Part model, mm, in its own coordinate system. Face numbers are marked on the shaded views. A direction names the side the tool comes from. Round coordinates to 2 decimals unless told otherwise and drop trailing zeros. Loops run counter-clockwise (first coordinate to the right, second up) from the corner with the lowest first, then second, coordinate; pieces in that order, holes last. Notation, with made-up numbers: (87, 34.25) - (124, 34.25) arc R29 cw to (124, 60.25) - close; hole circle Ø2 at (78.25, 28.5). An arc over 180 degrees is marked (long way). Write each question's results on one line, items separated by ' | '. Start each with the question number.
(1) Cut at D-D, the plane x = -40.5. List the corners of the cut face in (y, z) (3 decimals), then the cut area to 3 significant figures.
(2) Drill centre lines: L1, parallel to X at y = 23.5, z = 11; L2, parallel to Y at x = -29, z = 13.25; L3, parallel to X at y = -0.5, z = 14.25. Where is each one in solid material? Low to high.
(3) Mould opens along Y. For the marked faces 6, 7, 8 and 9 say: released by +Y, released by -Y, zero draft, split by the parting line, or undercut.
(4) Cut at B-B, the plane x = -24.5. List the corners of the cut face in (y, z).
(5) Cut at A-A, the plane y = 8. List the corners of the cut face in (x, z).
(6) Cut at C-C, the plane z = 16.5. List the corners of the cut face in (x, y), then the cut area to 3 significant figures.
(7) Tool access for the marked faces 1, 2, 3, 4 and 5: list every direction of +Z, -Z, +X, -X, +Y, -Y with a clear straight run to the whole face (end or side of a thin tool).
(8) Flat gauge pins, fed straight in: P1, Ø4, axis at x = -40.5, z = 17.5, coming from the +Y side; P2, Ø3, axis at x = -43.5, z = 11.5, coming from the -Y side; P3, Ø1.1, axis at x = 1.5, z = 13.5, coming from the -Y side; P4, Ø3, axis at y = 44, z = 11.5, coming from the +X side. Where does each tip first touch, or does it go through?
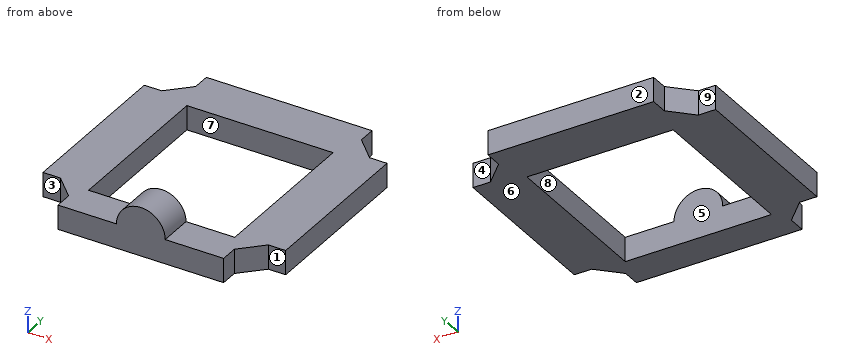
Autodesk Inventor part; units mm, degrees
ref_plane "Work Plane1" through (0, 0, 10) normal (0, 0, 1) x (1, 0, 0)
ref_plane "YZ Plane" through (0, 0, 0) normal (1, 0, 0) x (0, 1, 0)
ref_plane "XZ Plane" through (0, 0, 0) normal (0, 1, 0) x (-1, 0, 0)
ref_plane "Work Plane1" through (0, 0, 10) normal (0, 0, 1) x (1, 0, 0)
sketch "Sketch1" plane through (0, 0, 10) normal (0, 0, 1) x (1, 0, 0)
  line L0 (-4.0299, -0.3538) -> (-2.2322, 1.4439) construction
  arc A0 (-1.4439, 2.2322) -> (-2.2322, 1.4439) centre (-0.9299, 0.9299) ccw construction
  line L1 (-1.4439, 2.2322) -> (0.3538, 4.0299) construction
  line L2 (-37.8299, 42.2137) -> (-37.8299, 45.8299) construction
  line L3 (-37.8299, 45.8299) -> (-4.0299, 45.8299) construction
  line L4 (-4.0299, 45.8299) -> (-4.0299, 42.2137) construction
  line L5 (-4.0299, 4.0299) -> (0.3538, 4.0299)
  circle A1 centre (-20.9299, 20.9299) radius 17.5
  line L6 (-20.9299, 58.9723) -> (17.1124, 20.9299) construction
  line L7 (17.1124, 20.9299) -> (-20.9299, -17.1124) construction
  line L8 (-20.9299, -17.1124) -> (-58.9723, 20.9299) construction
  line L9 (-58.9723, 20.9299) -> (-20.9299, 58.9723) construction
  line L10 (-20.9299, 58.9723) -> (-20.9299, -17.1124) construction
  line L11 (17.1124, 20.9299) -> (-58.9723, 20.9299) construction
  line L12 (-20.9299, 58.9723) -> (32.8701, 58.9723) construction
  line L13 (-43.4299, 43.4299) -> (1.5701, 43.4299) construction
  line L14 (1.5701, 43.4299) -> (1.5701, -1.5701) construction
  line L15 (1.5701, -1.5701) -> (-43.4299, -1.5701) construction
  line L16 (-43.4299, -1.5701) -> (-43.4299, 43.4299) construction
  line L17 (-43.4299, 43.4299) -> (1.5701, -1.5701) construction
  line L18 (1.5701, 43.4299) -> (-43.4299, -1.5701) construction
  line L19 (-43.4299, 5.3876) -> (-43.4299, 36.4723)
  line L20 (-43.4299, 36.4723) -> (-36.4723, 43.4299)
  line L21 (-36.4723, 43.4299) -> (-5.3876, 43.4299)
  line L22 (-5.3876, 43.4299) -> (1.5701, 36.4723)
  line L23 (1.5701, 36.4723) -> (1.5701, 5.3876)
  line L24 (1.5701, 5.3876) -> (-5.3876, -1.5701)
  line L25 (-5.3876, -1.5701) -> (-36.4723, -1.5701)
  line L26 (-36.4723, -1.5701) -> (-43.4299, 5.3876)
  line L27 (-4.0299, 42.2137) -> (-37.8299, 42.2137)
  line L28 (-4.0299, -0.3538) -> (-4.0299, 4.0299)
  circle A2 centre (-20.9299, 20.9299) radius 0.4266
  point P0 (-37.8299, 4.0299)
  dimension "d18" = 53.8
  dimension "d19" = 45
  dimension "d20" = 53.8
  dimension "d21" = 45
  dimension "d22" = 45
extrude "Extrusion1" add sketch "Sketch1" along normal blind 5 contours L28 L24 L25 L26 L19 L20 L27 L22 L23 L5 | L5 L24 L28 | L27 L20 L21 L22 | A1
sketch "Sketch3" plane through (0, 0, 10) normal (0, 0, -1) x (-1, 0, 0)
  line L0 (37.8299, -0.4701) -> (37.8299, 4.0299) construction
  line L1 (4.0299, 4.0299) -> (4.0299, -0.4701) construction
  line L2 (37.8299, -0.4701) -> (37.8299, 1.1886) construction
  line L3 (4.0299, -3.9701) -> (4.0299, -0.3538) construction
  line L4 (45.8299, 4.0299) -> (42.2137, 4.0299) construction
  line L5 (-0.3538, 4.0299) -> (-3.9701, 4.0299) construction
  line L6 (-3.9701, 37.8299) -> (-0.3538, 37.8299) construction
  line L7 (4.0299, 42.2137) -> (4.0299, 45.8299) construction
  line L8 (37.8299, 45.8299) -> (37.8299, 42.2137) construction
  line L9 (42.2137, 37.8299) -> (45.8299, 37.8299) construction
  line L10 (37.8299, 37.7299) -> (45.8299, 37.7299)
  line L11 (45.8299, 37.7299) -> (45.8299, 4.1299)
  line L12 (45.8299, 4.1299) -> (37.8299, 4.1299)
  line L13 (37.8299, 4.1299) -> (37.8299, 37.7299)
  line L14 (37.7299, 4.0299) -> (4.1299, 4.0299)
  line L15 (4.1299, 4.0299) -> (4.1299, -3.9701)
  line L16 (4.1299, -3.9701) -> (37.7299, -3.9701)
  line L17 (37.7299, -3.9701) -> (37.7299, 4.0299)
  line L18 (4.0299, 4.1299) -> (-3.9701, 4.1299)
  line L19 (-3.9701, 4.1299) -> (-3.9701, 37.7299)
  line L20 (-3.9701, 37.7299) -> (4.0299, 37.7299)
  line L21 (4.0299, 37.7299) -> (4.0299, 4.1299)
  line L22 (4.1299, 37.8299) -> (37.7299, 37.8299)
  line L23 (37.7299, 37.8299) -> (37.7299, 45.8299)
  line L24 (37.7299, 45.8299) -> (4.1299, 45.8299)
  line L25 (4.1299, 45.8299) -> (4.1299, 37.8299)
  point P0 (0, 0)
  dimension "d23" = 0.1
  dimension "d24" = 0.1
  dimension "d25" = 0.1
  dimension "d26" = 0.1
  dimension "d27" = 0.1
extrude "Extrusion3" add sketch "Sketch3" against normal up to surface (5 mm away)
sketch "Skizze12" plane through (0, 0, 10) normal (0, 0, -1) x (-1, 0, 0)
  line L0 (-0.3124, 4.1299) -> (4.1299, -0.3124)
  line L1 (4.1299, -0.3124) -> (4.1299, -3.9701)
  line L2 (4.1299, -3.9701) -> (37.7299, -3.9701) construction
  line L3 (37.7299, -3.9701) -> (37.7299, -0.3124)
  line L4 (37.7299, -0.3124) -> (42.1723, 4.1299)
  line L5 (45.8299, 4.1299) -> (42.1723, 4.1299)
  line L6 (45.8299, 37.7299) -> (45.8299, 4.1299) construction
  line L7 (42.1723, 37.7299) -> (45.8299, 37.7299)
  line L8 (42.1723, 37.7299) -> (37.7299, 42.1723)
  line L9 (37.7299, 42.1723) -> (37.7299, 45.8299)
  line L10 (37.7299, 45.8299) -> (4.1299, 45.8299) construction
  line L11 (4.1299, 45.8299) -> (4.1299, 42.1723)
  line L12 (4.1299, 42.1723) -> (-0.3124, 37.7299)
  line L13 (-3.9701, 37.7299) -> (-0.3124, 37.7299)
  line L14 (-3.9701, 4.1299) -> (-3.9701, 37.7299) construction
  line L15 (-0.3124, 4.1299) -> (-3.9701, 4.1299)
  circle A0 centre (20.9299, 20.9299) radius 0.4266 construction
  line L16 (37.9299, -4.1701) -> (3.9299, -4.1701) construction
  line L17 (3.9299, -4.1701) -> (3.9299, -0.3953)
  line L18 (3.9299, -0.3953) -> (-0.3953, 3.9299)
  line L19 (-0.3953, 3.9299) -> (-4.1701, 3.9299)
  line L20 (-4.1701, 3.9299) -> (-4.1701, 37.9299) construction
  line L21 (-4.1701, 37.9299) -> (-0.3953, 37.9299)
  line L22 (-0.3953, 37.9299) -> (3.9299, 42.2551)
  line L23 (3.9299, 42.2551) -> (3.9299, 46.0299)
  line L24 (3.9299, 46.0299) -> (37.9299, 46.0299) construction
  line L25 (37.9299, 46.0299) -> (37.9299, 42.2551)
  line L26 (37.9299, 42.2551) -> (42.2551, 37.9299)
  line L27 (42.2551, 37.9299) -> (46.0299, 37.9299)
  line L28 (46.0299, 37.9299) -> (46.0299, 3.9299) construction
  line L29 (46.0299, 3.9299) -> (42.2551, 3.9299)
  line L30 (42.2551, 3.9299) -> (37.9299, -0.3953)
  line L31 (37.9299, -0.3953) -> (37.9299, -4.1701)
  line L32 (-3.9701, 37.7299) -> (-3.9701, 37.9299)
  line L33 (37.7299, 45.8299) -> (4.1299, 45.8299)
  line L34 (4.1299, 45.8299) -> (3.9299, 45.8299)
  line L35 (37.7299, 45.8299) -> (37.9299, 45.8299)
  line L36 (45.8299, 37.7299) -> (45.8299, 37.9299)
  line L37 (45.8299, 4.1299) -> (45.8299, 3.9299)
  line L38 (37.7299, -3.9701) -> (37.9299, -3.9701)
  line L39 (4.1299, -3.9701) -> (3.9299, -3.9701)
  line L40 (-3.9701, 4.1299) -> (-3.9701, 3.9299)
  point P0 (0, 0)
  dimension "d65" = 0.2
extrude "IM_offset" add sketch "Skizze12" against normal up to surface (5 mm away)
ref_plane "Work Plane4" through (-37.9299, 6.0299, 10) normal (0, -1, 0) x (1, 0, 0)
sketch "Sketch17" plane through (-37.9299, 6.0299, 10) normal (0, -1, 0) x (1, 0, 0)
  line L0 (0, 5) -> (34, 5)
  line L1 (34, 0) -> (34, 5)
  line L2 (0, 0) -> (34, 0)
  line L3 (0, 0) -> (0, 5)
  line L4 (17.4266, 0) -> (16.5734, 0)
  line L5 (16.5734, 5) -> (17.4266, 5)
  line L6 (17.4266, 0) -> (16.5734, 0)
  line L7 (32, 5) -> (2, 5)
  line L8 (2, 5) -> (2, 0)
  line L9 (2, 0) -> (32, 0)
  line L10 (32, 0) -> (32, 5)
  line L11 (32, 5) -> (2, 0) construction
  line L12 (2, 5) -> (32, 0) construction
  point P0 (37.9299, -10)
  point P1 (17, 2.5)
  dimension "d91" = 30
extrude "Extrusion15" cut sketch "Sketch17" along normal blind 3 and the other way blind 30 contours L0 L10 L2 L8
sketch "Sketch18" plane through (-37.9299, 3.0299, 10) normal (0, -1, 0) x (1, 0, 0)
  line L0 (0, 5) -> (34, 5)
  line L1 (34, 0) -> (34, 5)
  line L2 (0, 0) -> (34, 0)
  line L3 (0, 0) -> (0, 5)
  line L4 (2, 5) -> (32, 5)
  circle A0 centre (17, 5) radius 5
  point P0 (37.9299, -10)
  point P1 (32, -5)
  point P2 (2, -5)
extrude "Extrusion16" add sketch "Sketch18" along normal up to surface (7 mm away) contours A0 L0 | L0 A0
properties part number "20_Cube_Insert_Despeckler_upright_motor_v3"
A:
1) outline: (2.175, 10) - (39.685, 10) - (39.685, 15) - (2.175, 15) - close | area: 188 mm2
2) L1: -45.83 to -35.93, -5.93 to 3.97 | L2: -3.97 to 3.03, 36.03 to 45.83 | L3: -37.93 to -3.93
3) face 6: zero draft | face 7: undercut | face 8: undercut | face 9: released by +Y
4) outline: (-3.97, 10) - (3.03, 10) - (3.03, 18.5) - (-3.97, 18.5) - close; (36.03, 10) - (45.83, 10) - (45.83, 15) - (36.03, 15) - close
5) outline: (-45.83, 10) - (-35.93, 10) - (-35.93, 15) - (-45.83, 15) - close; (-5.93, 10) - (3.97, 10) - (3.97, 15) - (-5.93, 15) - close
6) outline: (-25.7, -3.97) - (-16.16, -3.97) - (-16.16, 3.03) - (-25.7, 3.03) - close | area: 66.8 mm2
7) face 1: +Z, -Z, +X, -Y | face 2: +Z, -Z, +X, -X, +Y | face 3: +Z, -Z, -X, -Y | face 4: +Z, -Z, +X, +Y | face 5: +Z, -Z
8) P1: through | P2: y = 3.67 | P3: y = 3.93 | P4: x = -3.93
